Check sheet for the modelled part. Datum: model origin and axes. Units: mm. A direction names the side the tool comes from. Coordinates: 2 decimals unless noted, no trailing zeros. Loops run counter-clockwise (first coordinate to the right, second up) from the corner with the lowest first, then second, coordinate; pieces in that order, holes last. Notation, with made-up numbers: (40.25, 70) -> (57.25, 70) arc R21 cw to (57.25, 105) -> close; hole circle Ø11 at (-3, 6). An arc over 180 degrees is marked (long way). Use CSV: the item, a comma, the result in double quotes.
Autodesk Inventor part; units mm, degrees
ref_plane "YZ Plane" through (0, 0, 0) normal (1, 0, 0) x (0, 1, 0)
ref_plane "XZ Plane" through (0, 0, 0) normal (0, 1, 0) x (-1, 0, 0)
ref_plane "XY Plane" through (0, 0, 0) normal (0, 0, 1) x (1, 0, 0)
sketch "Sketch1" plane through (0, 0, 0) normal (0, 0, 1) x (1, 0, 0)
  circle A0 centre (0, 0) radius 4.5
  dimension "d0" = 9
extrude "Extrusion1" add sketch "Sketch1" along normal blind 10
ref_plane "Work Plane2" through (0, 0, 7.5) normal (0, 0, 1) x (1, 0, 0)
ref_plane "Work Plane1" through (0, 0, 5) normal (0, 0, 1) x (1, 0, 0)
sketch "Sketch2" plane through (0, 0, 7.5) normal (0, 0, 1) x (1, 0, 0)
  circle A0 centre (0, 0) radius 4.5
  circle A1 centre (0, 0) radius 2.75
  dimension "d3" = 5.5
  dimension "d4" = 9
extrude "Extrusion2" cut sketch "Sketch2" along normal mid plane 2
mirror "Mirror1" about plane through (0, 0, 5) normal (0, 0, 1) of "Extrusion2"
sketch "Sketch3" plane through (0, 0, 0) normal (0, 0, -1) x (-1, 0, 0)
  point P0 (0, 0)
sketch "Sketch4" plane through (0, 0, 0) normal (0, 0, -1) x (-1, 0, 0)
  circle A0 centre (0, 0) radius 1.8
  dimension "d11" = 3.6
extrude "Extrusion3" cut sketch "Sketch4" against normal blind 10
sketch "Sketch5" plane through (0, 0, 10) normal (0, 0, 1) x (1, 0, 0)
  circle A0 centre (0, 3.2193) radius 0.5
  point P0 (0, 0)
  dimension "d14" = 1
extrude "Extrusion4" cut sketch "Sketch5" against normal blind 10
properties part number "MotorPully"
1) Go/stop test with flat-tipped pins: pin 1 Ø5 at (x, z) = (-3, 3) entering from +Y; pin 2 Ø3 at (x, z) = (-3.5, 8.5) entering from -Y. Record where each tip stops, or that it passes through.
Answer below:
pin 1,"stops at y = 4.47"
pin 2,"stops at y = -4.03"
2) Cross-section at B-B on y = 4.25. Record the boundary of the cut face in (x, z), and give its area (3 significant figures).
Answer below:
outline,"(-1.48, 0) -> (1.48, 0) -> (1.48, 1.5) -> (-1.48, 1.5) -> close; (-1.48, 3.5) -> (1.48, 3.5) -> (1.48, 6.5) -> (-1.48, 6.5) -> close; (-1.48, 8.5) -> (1.48, 8.5) -> (1.48, 10) -> (-1.48, 10) -> close"
area,"17.7 mm²"
3) Thickness scan on line 1 along Z through (x, y) = (-0.25, -3.5); line 2 along Y through (x, z) = (0, 6); line 3 along Y through (x, z) = (0.25, 9). Record the ranges inside material, lowest first. Write a range as from..to.
Answer below:
line 1,"z = 0..1.5, 3.5..6.5, 8.5..10"
line 2,"y = -4.5..-1.8, 1.8..2.72, 3.72..4.5"
line 3,"y = -4.49..-1.78, 1.78..2.79, 3.65..4.49"
4) Cross-section at D-D on x = 2. Record the boundary of the cut face in (y, z).
Answer below:
outline,"(-4.03, 0) -> (4.03, 0) -> (4.03, 1.5) -> (1.89, 1.5) -> (1.89, 3.5) -> (4.03, 3.5) -> (4.03, 6.5) -> (1.89, 6.5) -> (1.89, 8.5) -> (4.03, 8.5) -> (4.03, 10) -> (-4.03, 10) -> (-4.03, 8.5) -> (-1.89, 8.5) -> (-1.89, 6.5) -> (-4.03, 6.5) -> (-4.03, 3.5) -> (-1.89, 3.5) -> (-1.89, 1.5) -> (-4.03, 1.5) -> close"
5) Draft check along Z on faces 3 (the cylindrical face through (-0.11, 2.73, 5.07)), 4 (the flat face through (0, -3, 1.5)), 5 (the flat face through (0, -3, 8.5)), 6 (the flat face through (0, -2, 10)). Enter one of: released by +Z, released by -Z, zero draft, split by the parting line, or undercut.
Answer below:
face 3,"zero draft"
face 4,"undercut"
face 5,"undercut"
face 6,"released by +Z"
6) Cross-section at A-A on x = 0. Record the boundary of the cut face in (y, z), and give its area (3 significant figures).
Answer below:
outline,"(-4.5, 0) -> (-1.8, 0) -> (-1.8, 10) -> (-4.5, 10) -> (-4.5, 8.5) -> (-2.75, 8.5) -> (-2.75, 6.5) -> (-4.5, 6.5) -> (-4.5, 3.5) -> (-2.75, 3.5) -> (-2.75, 1.5) -> (-4.5, 1.5) -> close; (1.8, 0) -> (2.72, 0) -> (2.72, 10) -> (1.8, 10) -> close; (3.72, 0) -> (4.5, 0) -> (4.5, 1.5) -> (3.72, 1.5) -> close; (3.72, 3.5) -> (4.5, 3.5) -> (4.5, 6.5) -> (3.72, 6.5) -> close; (3.72, 8.5) -> (4.5, 8.5) -> (4.5, 10) -> (3.72, 10) -> close"
area,"33.9 mm²"
7) Cross-section at C-C on y = -1.25. Record the boundary of the cut face in (x, z).
Answer below:
outline,"(-4.32, 0) -> (-1.3, 0) -> (-1.3, 10) -> (-4.32, 10) -> (-4.32, 8.5) -> (-2.45, 8.5) -> (-2.45, 6.5) -> (-4.32, 6.5) -> (-4.32, 3.5) -> (-2.45, 3.5) -> (-2.45, 1.5) -> (-4.32, 1.5) -> close; (1.3, 0) -> (4.32, 0) -> (4.32, 1.5) -> (2.45, 1.5) -> (2.45, 3.5) -> (4.32, 3.5) -> (4.32, 6.5) -> (2.45, 6.5) -> (2.45, 8.5) -> (4.32, 8.5) -> (4.32, 10) -> (1.3, 10) -> close"
8) Access from +Z, -Z, +X, -X, +Y, -Y to the whole of each face (thin tool, end or side, straight path). Record for faces 1 (the flat face through (0, -3, 6.5)), 2 (the cylindrical face through (-0.59, -4.46, 4.98)).
Answer below:
face 1,"none"
face 2,"+Z, -Z"
